Print and shaded views of the part. All mm, measured from the part's lowest x, y and z. Give positions to 0.01 mm unless a question says otherwise; leave off trailing zeros. Loops run counter-clockwise (first coordinate to the right, second up) from the corner with the lowest first, then second, coordinate; pieces in that order, holes last. Notation, with made-up numbers: (54.25, 33.25) - (61.25, 33.25) arc R9 ccw to (61.25, 43.25) - close; hole circle Ø6 at (73, 84). An arc over 180 degrees is marked (long way). Return JSON: item names as keys, results as strings.
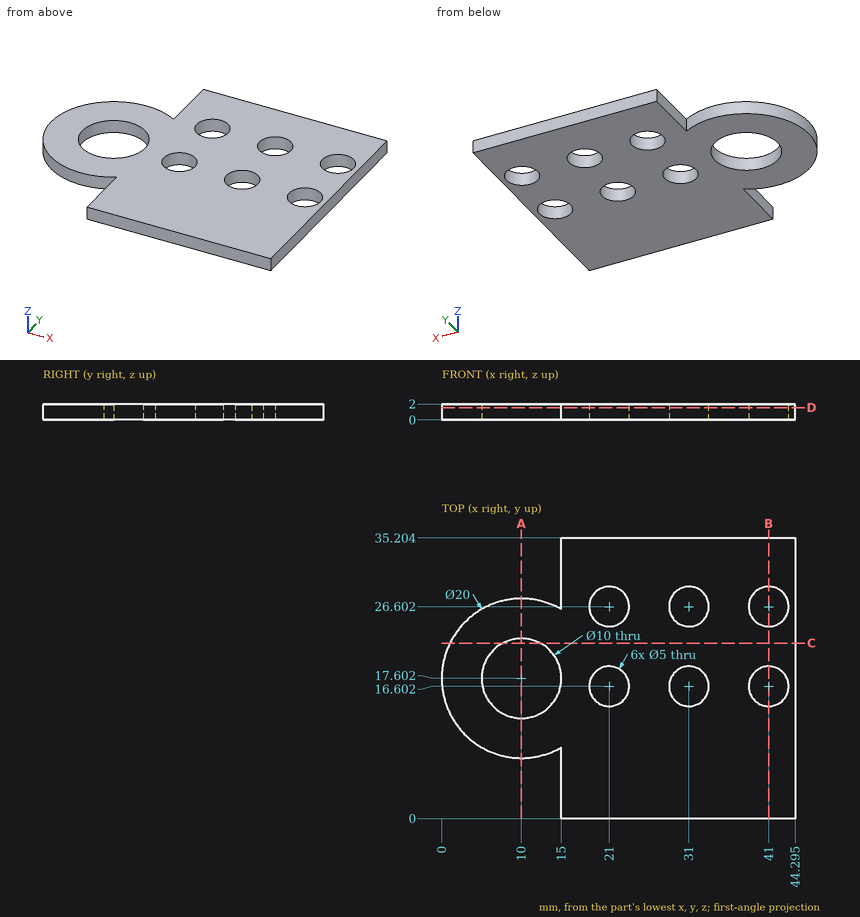
1. Cut at C-C, the plane y = 22. Write the cut outline in (x, z) (1 decimal).
Values follow:
{"outline": "(1, 0) - (7.6, 0) - (7.6, 2) - (1, 2) - close; (12.4, 0) - (44.3, 0) - (44.3, 2) - (12.4, 2) - close"}
2. Cut at A-A, the plane x = 10. Write the cut outline in (y, z), plus the area to 3 significant figures.
Values follow:
{"outline": "(7.6, 0) - (12.6, 0) - (12.6, 2) - (7.6, 2) - close; (22.6, 0) - (27.6, 0) - (27.6, 2) - (22.6, 2) - close", "area": "20.0 mm²"}
3. Drill centre lines: probe 1 along Y at (x, z) = (21, 1.2); probe 2 along Y at (x, z) = (19, 0.55) (1 decimal); probe 3 along X at (y, z) = (17, 1.4) (1 decimal). Where is each one in solid material? Low to high.
Values follow:
{"probe 1": "y = 0 to 14.1, 19.1 to 24.1, 29.1 to 35.2", "probe 2": "y = 0 to 15.1, 18.1 to 25.1, 28.1 to 35.2", "probe 3": "x = 0 to 5, 15 to 18.5, 23.5 to 28.5, 33.5 to 38.5, 43.5 to 44.3"}
4. Cut at B-B, the plane x = 41. Write the cut outline in (y, z), plus the area to 3 significant figures.
Values follow:
{"outline": "(0, 0) - (14.1, 0) - (14.1, 2) - (0, 2) - close; (19.1, 0) - (24.1, 0) - (24.1, 2) - (19.1, 2) - close; (29.1, 0) - (35.2, 0) - (35.2, 2) - (29.1, 2) - close", "area": "50.4 mm²"}
5. Cut at D-D, the plane z = 1.55. Write the cut outline in (x, y) (1 decimal), plus the area to 3 significant figures.
Values follow:
{"outline": "(15, 0) - (44.3, 0) - (44.3, 35.2) - (15, 35.2) - (15, 26.3) arc R10 ccw (long way) to (15, 8.9) - close; hole circle Ø10 at (10, 17.6); hole circle Ø5 at (21, 16.6); hole circle Ø5 at (21, 26.6); hole circle Ø5 at (31, 16.6); hole circle Ø5 at (31, 26.6); hole circle Ø5 at (41, 16.6); hole circle Ø5 at (41, 26.6)", "area": "1,090 mm²"}
